Autodesk Inventor part; units mm, degrees
ref_plane "tnut_XY" through (0, 4.3434, 0) normal (0, 1, 0) x (1, 0, 0)
ref_plane "tnut_YZ" through (0, 4.3434, 0) normal (1, 0, 0) x (0, 0, -1)
ref_plane "tnut_ZX" through (0, 4.3434, 0) normal (0, 0, -1) x (0, 1, 0)
sketch "Sketch_1" plane through (0, 0, -7.366) normal (0, 0, 1) x (1, 0, 0)
  line L0 (-5.4737, 3.9624) -> (-5.4737, 2.5467)
  arc A0 (-5.4737, 2.5467) -> (-5.3621, 2.2773) centre (-5.0927, 2.5467) ccw
  line L1 (-5.3621, 2.2773) -> (-3.1964, 0.1116)
  arc A1 (-3.1964, 0.1116) -> (-2.927, 0) centre (-2.927, 0.381) ccw
  line L2 (-2.927, 0) -> (2.927, 0)
  arc A2 (2.927, 0) -> (3.1964, 0.1116) centre (2.927, 0.381) ccw
  line L3 (3.1964, 0.1116) -> (5.3621, 2.2773)
  arc A3 (5.3621, 2.2773) -> (5.4737, 2.5467) centre (5.0927, 2.5467) ccw
  line L4 (5.4737, 2.5467) -> (5.4737, 3.9624)
  arc A4 (5.4737, 3.9624) -> (5.0927, 4.3434) centre (5.0927, 3.9624) ccw
  line L5 (5.0927, 4.3434) -> (-5.0927, 4.3434)
  arc A5 (-5.0927, 4.3434) -> (-5.4737, 3.9624) centre (-5.0927, 3.9624) ccw
extrude "Extrusion1" add sketch "Sketch_1" along normal blind 12.446
sketch "Sketch_3" plane through (0, 0, 0) normal (0, 0, 1) x (1, 0, 0)
  line L0 (0, 0) -> (0, 4.3434)
  line L1 (0, 4.3434) -> (3.175, 4.3434)
  line L2 (3.175, 4.3434) -> (2.4879, 3.6563)
  line L3 (2.4879, 3.6563) -> (2.4879, 0.6871)
  line L4 (2.4879, 0.6871) -> (3.175, 0)
  line L5 (3.175, 0) -> (0, 0)
  line L6 (0, 0) -> (0, 4.3434)
revolve "Revolution1" cut sketch "Sketch_3" angle 360 about axis through (0, 0, 0) along (0, -1, 0)
thread "Thread1"
ref_plane "tnut_XY" through (0, 4.3434, 0) normal (0, 1, 0) x (1, 0, 0)
ref_plane "tnut_YZ" through (0, 4.3434, 0) normal (1, 0, 0) x (0, 0, -1)
ref_plane "tnut_ZX" through (0, 4.3434, 0) normal (0, 0, -1) x (0, 1, 0)
properties part number "3204"
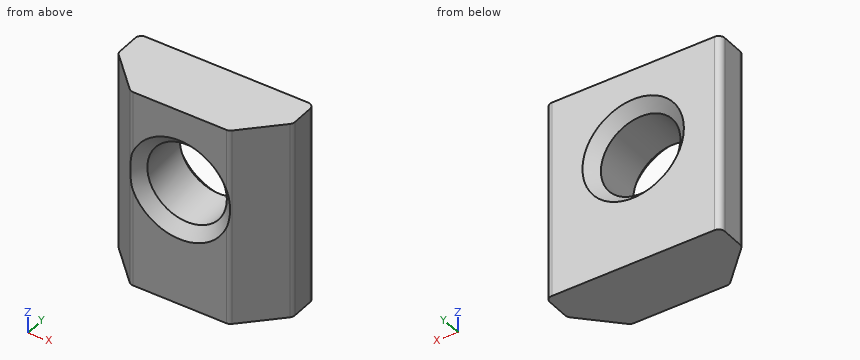
Geometry check sheet. Reference: the model listing, model coordinates, mm. Round coordinates to 2 decimals unless told otherwise and drop trailing zeros. Order: outer loops, then holes, each group sorted by start corner. A loop starts at its lowest first (then second) coordinate and runs counter-clockwise, first axis right, second up. Notation, with made-up numbers: (49.25, 86.5) -> (96.25, 86.5) arc R21 ccw to (96.25, 91.5) -> close; hole circle Ø9 at (-36, 71.25). An arc over 180 degrees is marked (long way). Return JSON: item names as keys, results as strings. Group by question number.
Q1. Section check B-B, the plane x = 0. Record the boundary of the cut face in (y, z) (3 decimals).
Q2. Material ranges on probe 1 along Z at (x, y) = (0, 2.5); probe 2 along X at (y, z) = (0.8, -1.25); probe 3 along Z at (x, y) = (-1.25, 3), recorded low to high. Write a range as from..to.
Q3. Section check A-A, the plane z = 4. Record the boundary of the cut face in (x, y), plus the area to 3 significant figures.
Q4. Section check C-C, the plane y = 3.2. Record the boundary of the cut face in (x, z).
Q5. Section check D-D, the plane z = 0. Record the boundary of the cut face in (x, y) (3 decimals), plus the area to 3 significant figures.
Numbers:
{
 "1": {"outline": "(0, -7.366) -> (4.343, -7.366) -> (4.343, -3.175) -> (3.656, -2.488) -> (0.687, -2.488) -> (0, -3.175) -> close; (0, 3.175) -> (0.687, 2.488) -> (3.656, 2.488) -> (4.343, 3.175) -> (4.343, 5.08) -> (0, 5.08) -> close"},
 "2": {"probe 1": "-7.37..-2.49, 2.49..5.08", "probe 2": "-3.88..-2.15, 2.15..3.88", "probe 3": "-7.37..-2.15, 2.15..5.08"},
 "3": {"outline": "(-5.47, 2.55) arc R0.38 ccw to (-5.36, 2.28) -> (-3.2, 0.11) arc R0.38 ccw to (-2.93, 0) -> (2.93, 0) arc R0.38 ccw to (3.2, 0.11) -> (5.36, 2.28) arc R0.38 ccw to (5.47, 2.55) -> (5.47, 3.96) arc R0.38 ccw to (5.09, 4.34) -> (-5.09, 4.34) arc R0.38 ccw to (-5.47, 3.96) -> close", "area": "41.8 mm^2"},
 "4": {"outline": "(-5.47, -7.37) -> (5.47, -7.37) -> (5.47, 5.08) -> (-5.47, 5.08) -> close; hole circle Ø4.98 at (0, 0)"},
 "5": {"outline": "(-5.474, 2.547) arc R0.381 ccw to (-5.362, 2.277) -> (-3.196, 0.112) arc R0.381 ccw to (-3.122, 0.053) -> (-2.488, 0.687) -> (-2.488, 3.656) -> (-3.175, 4.343) -> (-5.093, 4.343) arc R0.381 ccw to (-5.474, 3.962) -> close; (2.488, 0.687) -> (3.122, 0.053) arc R0.381 ccw to (3.196, 0.112) -> (5.362, 2.277) arc R0.381 ccw to (5.474, 2.547) -> (5.474, 3.962) arc R0.381 ccw to (5.093, 4.343) -> (3.175, 4.343) -> (2.488, 3.656) -> close", "area": "19.2 mm^2"}
}
